Here's how the part is built. I have some questions about the finished solid (model axes, mm). Face numbers are marked on the shaded views. A direction names the side the tool comes from. Give positions to 0.01 mm unless a question says otherwise; leave off trailing zeros. Write each loop counter-clockwise with the first axis right and the second up, starting at its lowest first coordinate (ties: lowest second). Pieces come first, ordered by that corner, then holes. Notation, with made-up numbers: (64, 54.5) -> (107, 54.5) arc R11 cw to (107, 63.5) -> close; hole circle Ø5 at (53, 4.25). An arc over 180 degrees is marked (long way). Return JSON: item names as keys, results as strings.
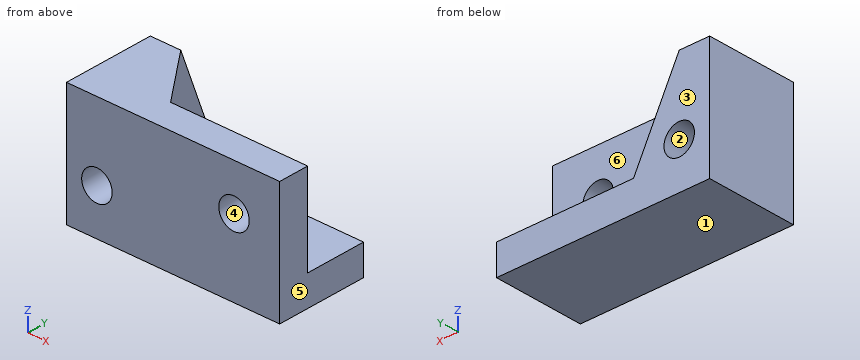
from build123d import *

# Parameters (mm, degrees)
SKETCH1_W           = 70
SKETCH1_H           = 40
BOSS_EXTRUDE1_DEPTH = 30
SKETCH2_W           = 30
SKETCH2_H           = 20
CUT_EXTRUDE1_DEPTH  = 30
CUT_EXTRUDE2_DEPTH  = 36
CUT_EXTRUDE3_DEPTH  = 49
CUT_EXTRUDE5_DEPTH  = 21
SKETCH11_R          = 5
CUT_EXTRUDE6_DEPTH  = 11
SKETCH12_R          = 5
CUT_EXTRUDE7_DEPTH  = 31


with BuildPart() as part:
    # Sketch1 → Boss-Extrude1 (new body)
    with BuildSketch(Plane(origin=(0, 0, 0), x_dir=(1, 0, 0), z_dir=(0, 1, 0))):
        with Locations((35, 20)):
            Rectangle(SKETCH1_W, SKETCH1_H)
    extrude(amount=BOSS_EXTRUDE1_DEPTH)

    # Sketch2 → Cut-Extrude1 (cut)
    with BuildSketch(Plane.XY):
        with Locations((55, 20)):
            Rectangle(SKETCH2_W, SKETCH2_H)
    extrude(amount=-CUT_EXTRUDE1_DEPTH, mode=Mode.SUBTRACT)

    # Sketch8 → Cut-Extrude2 (cut)
    with BuildSketch(Plane(origin=(17.931034483, 13.448275862, 8.965517241), x_dir=(0.297112541, 0.222834406, -0.928476691), z_dir=(0.742781353, 0.557086015, 0.371390676))):
        Polygon((9.656157585, 18), (9.656157585, -7), (41.967146428, -16), (41.967146428, 9), align=None)
    extrude(amount=CUT_EXTRUDE2_DEPTH, mode=Mode.SUBTRACT)

    # Sketch9 → Cut-Extrude3 (cut)
    with BuildSketch(Plane.XY.offset(-30)):
        Polygon((25, 30), (40, 10), (40, 30), align=None)
    extrude(amount=CUT_EXTRUDE3_DEPTH, mode=Mode.SUBTRACT)

    # Sketch10 → Cut-Extrude5 (cut)
    with BuildSketch(Plane(origin=(0, 10, 0), x_dir=(1, 0, 0), z_dir=(0, 1, 0))):
        Polygon((25, 0), (40, 0), (40, 30), align=None)
    extrude(amount=CUT_EXTRUDE5_DEPTH, mode=Mode.SUBTRACT)

    # Sketch11 → Cut-Extrude6 (cut, through all)
    with BuildSketch(Plane(origin=(0, 10, 0), x_dir=(1, 0, 0), z_dir=(0, 1, 0))):
        with Locations((55, 15)):
            Circle(SKETCH11_R)
    extrude(amount=-CUT_EXTRUDE6_DEPTH, mode=Mode.SUBTRACT)

    # Sketch12 → Cut-Extrude7 (cut, through all)
    with BuildSketch(Plane(origin=(0, 30, 0), x_dir=(1, 0, 0), z_dir=(0, 1, 0))):
        with Locations((10, 25)):
            Circle(SKETCH12_R)
    extrude(amount=-CUT_EXTRUDE7_DEPTH, mode=Mode.SUBTRACT)


solid = part.part
1. For pin 1 Ø6 at (x, y) = (41.5, 23.5) entering from +Z; pin 2 Ø15 at (x, z) = (51, -16.5) entering from +Y; pin 3 Ø3 at (y, z) = (16.5, -7) entering from +X, each with a flat end and sliding along its axis, tell me the tip position at first contact or that it passes through.
Taken from the geometry:
{"pin 1": "stops at z = -30", "pin 2": "stops at y = 10", "pin 3": "stops at x = 24.98"}
2. Which directions (+Z, -Z, +X, -X, +Y, -Y) give clear straight access to the entire face, cutting with the end or side of a thin tool? Please do the marked faces 5 and 6.
Taken from the geometry:
{"face 5": "+Z, -Z, +X, +Y, -Y", "face 6": "+Z, +X, +Y"}
3. If I drill on line 1 (X direction, y = 7, z = -15); line 2 (Z direction, x = 55, y = 6.25); line 3 (Y direction, x = 65.5, z = -13.5), over which ranges is the centre line in solid material (lowest first)? Write a range as [from, to].
Taken from the geometry:
{"line 1": "x = [0, 50], [60, 70]", "line 2": "z = [-40, -20], [-10, 0]", "line 3": "y = [0, 10]"}
4. If we mould it in two halves opening along Z, with no side actions, what happens to the marked faces 1, 2, 3 and 4? For each: released by +Z, released by -Z, zero draft, split by the parting line, or undercut.
Taken from the geometry:
{"face 1": "released by -Z", "face 2": "undercut", "face 3": "zero draft", "face 4": "undercut"}
5. Suppose I cut it at C-C, the plane x = 32.5. List the corners of the cut face in (y, z) for me.
Taken from the geometry:
{"outline": "(0, -40) -> (30, -40) -> (30, -30) -> (20, -30) -> (10, -15) -> (10, 0) -> (0, 0) -> close"}
6. Suppose I cut it at D-D, the plane y = 25.5. List the corners of the cut face in (x, z) for me (3 decimals).
Taken from the geometry:
{"outline": "(0, -40) -> (70, -40) -> (70, -30) -> (28.375, -30) -> (13.375, 0) -> (0, 0) -> close; hole circle Ø10 at (10, -25)"}
7. Suppose I cut it at B-B, the plane x = 55. List the corners of the cut face in (y, z) for me, and give its area (3 significant figures).
Taken from the geometry:
{"outline": "(0, -40) -> (30, -40) -> (30, -30) -> (10, -30) -> (10, -20) -> (0, -20) -> close; (0, -10) -> (10, -10) -> (10, 0) -> (0, 0) -> close", "area": "500 mm²"}
8. Suppose I cut it at A-A, the plane z = -25. List the corners of the cut face in (x, y) for me, and give its area (4 significant figures).
Taken from the geometry:
{"outline": "(0, 0) -> (5, 0) -> (5, 30) -> (0, 30) -> close; (15, 0) -> (70, 0) -> (70, 10) -> (37.5, 10) -> (22.5, 30) -> (15, 30) -> close", "area": "1,000 mm²"}
